```python
from build123d import *

# Parameters (mm, degrees)
F1_DEPTH = 50.8
F2_R     = 5.07999
F3_R     = 2.6971074435
F4_DEPTH = 25.4


# Not quite as in the source:
# - a fillet or chamfer is up to 0.001 mm smaller than in the source, because OpenCascade refuses the exact size


with BuildPart() as f1:
    # F0 (on Top) → F1 (new body)
    with BuildSketch(Plane.XY):
        Polygon((-30.48, 1.27), (-30.48, 5.08), (30.48, 5.08), (30.48, -5.08), (-30.48, -5.08), (-35.56, -5.08), (-35.56, -10.16), (35.56, -10.16), (35.56, 10.16), (-35.56, 10.16), (-35.56, 1.27), align=None)
    extrude(amount=F1_DEPTH)

    # F2 (radius 5.08 in the source; OpenCascade refuses exactly that, so slightly less here)
    f2_edges = [f1.edges().sort_by_distance(p)[0] for p in [
        (35.56, 10.16, 25.4),
        (35.56, -10.16, 25.4),
        (-35.56, 10.16, 25.4),
        (-35.56, -10.16, 25.4),
    ]]
    fillet(f2_edges, radius=F2_R)

    # F3 (on face) → F4 (cut)
    with BuildSketch(Plane.XZ.offset(10.16)):
        with Locations((0, 25.9590707719)):
            Circle(F3_R)
    extrude(amount=-F4_DEPTH, mode=Mode.SUBTRACT)


solid = f1.part
```
Check sheet for the modelled part. Datum: model origin and axes. Units: mm. A direction names the side the tool comes from. Round coordinates to 2 decimals unless told otherwise and drop trailing zeros. Loops run counter-clockwise (first coordinate to the right, second up) from the corner with the lowest first, then second, coordinate; pieces in that order, holes last. Notation, with made-up numbers: (-33.5, -29) -> (-6.5, -29) arc R23 ccw to (-6.5, -18) -> close; hole circle Ø6 at (1, -26). An arc over 180 degrees is marked (long way). Write item = value, one per line. Start each with the question number.
1) Set-up check for faces 1 (the cylindrical face through (-34.111, -8.632, 25.756)), 2 (the flat face through (-33, 1.27, 25)), 3 (the flat face through (0, 5.08, 31)): record each of +Z, -Z, +X, -X, +Y, -Y from which the full face is reachable in a straight line by a thin tool's end or side.
2) Sectioned sample at C-C, the plane y = -7.25. Record the cut outline in (x, z).
3) Thickness scan on probe 1 along Y at (x, z) = (-12, 15); probe 2 along Z at (x, y) = (0, 7.75); probe 3 along X at (y, z) = (3.5, 46.5). Record the ranges inside material, lowest first.
4) Release check for a two-part mould opening along Z. For faces 4 (the cylindrical face through (-0.351, -7.656, 28.633)), 5 (the flat face through (-30.48, 3, 25)), 6 (the flat face through (0, 7, 50.8)) record: released by +Z, released by -Z, zero draft, split by the parting line, or undercut.
5) Sectioned sample at D-D, the plane y = 9. Record the cut outline in (x, z), plus the area to 3 significant figures.
6) Sectioned sample at A-A, the plane x = -7. Record the cut outline in (y, z).
7) Gauge pin test, flat end, axial feed: pin 1 Ø3 at (y, z) = (7, 30.5) entering from +X. Record the tip position at first contact, or that the pin passes through.
Results are:
q1.face_1 = +Z, -Z, -X, -Y
q1.face_2 = +Z, -Z, -X
q1.face_3 = +Z, -Z
q2.outline = (-35.07, 0) -> (35.07, 0) -> (35.07, 50.8) -> (-35.07, 50.8) -> close; hole circle Ø5.39 at (0, 25.96)
q3.probe_1 = -10.16 to -5.08, 5.08 to 10.16
q3.probe_2 = 0 to 23.26, 28.66 to 50.8
q3.probe_3 = -35.56 to -30.48, 30.48 to 35.56
q4.face_4 = undercut
q4.face_5 = zero draft
q4.face_6 = released by +Z
q5.outline = (-33.71, 0) -> (33.71, 0) -> (33.71, 50.8) -> (-33.71, 50.8) -> close; hole circle Ø5.39 at (0, 25.96)
q5.area = 3,400 mm^2
q6.outline = (-10.16, 0) -> (-5.08, 0) -> (-5.08, 50.8) -> (-10.16, 50.8) -> close; (5.08, 0) -> (10.16, 0) -> (10.16, 50.8) -> (5.08, 50.8) -> close
q7.pin_1 = 35.54
